Can you work these out from the drawing? Everything is in mm from the part's minimum corner. A direction names the side the tool comes from. Coordinates: 2 decimals unless noted, no trailing zeros. Order: outer loops, then holes, each group sorted by start corner. A loop starts at its lowest first (then second) coordinate and runs counter-clockwise, first axis right, second up. Notation, with made-up numbers: (-28.5, 0) - (23.5, 0) arc R24 ccw to (23.5, 13) - close; hole circle Ø10 at (-3.5, 9.5). An arc over 180 degrees is marked (long way). One line per item, written item: value.
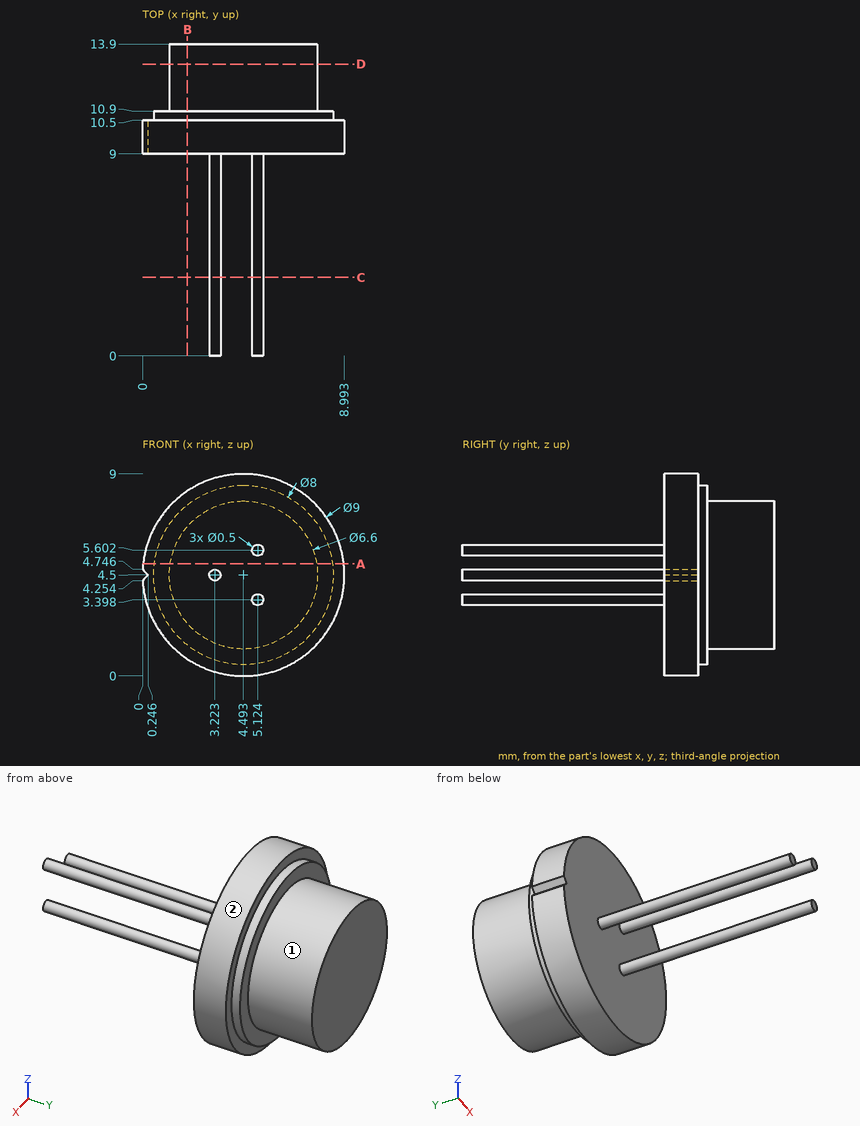
Item 1: For the marked faces 1 and 2, which set-ups out of +Z, -Z, +X, -X, +Y, -Y let a thin tool reach every point of the face, with its end or its side?
Conclusion:
face 1: +Y
face 2: +Y, -Y
Item 2: I want a section at C-C on y = 3.5. Please give me the cut outline in (x, z).
Conclusion:
outline: circle Ø0.5 at (3.22, 4.5); circle Ø0.5 at (5.12, 3.4); circle Ø0.5 at (5.12, 5.6)
Item 3: I want a section at D-D on y = 13. Please give me the cut outline in (x, z).
Conclusion:
outline: circle Ø6.6 at (4.49, 4.5)
Item 4: I want a section at A-A on z = 5. Please give me the cut outline in (x, y) (1 decimal).
Conclusion:
outline: (0, 9) - (9, 9) - (9, 10.5) - (8.5, 10.5) - (8.5, 10.9) - (7.8, 10.9) - (7.8, 13.9) - (1.2, 13.9) - (1.2, 10.9) - (0.5, 10.9) - (0.5, 10.5) - (0, 10.5) - close
Item 5: If I drill on probe 1 along Y at (x, z) = (3.5, 4.75); probe 2 along Y at (x, z) = (3.75, 0.5); probe 3 along Z at (x, y) = (5, 8) (1 decimal), over which ranges is the centre line in solid material (lowest first)?
Conclusion:
probe 1: 9 to 13.9
probe 2: 9 to 10.5
probe 3: 3.2 to 3.6, 5.4 to 5.8
Item 6: I'm going to push flat-ended pins straight in: pin 1 Ø5 at (x, z) = (1.5, 6.5) entering from -Y; pin 2 Ø1 at (x, z) = (7.5, 1.5) entering from +Y; pin 3 Ø1.5 at (y, z) = (2, 8) entering from -X; pin 4 Ø2 at (x, y) = (4.5, 4.5) entering from +Z. Where does each tip first touch, or does it pass through?
Conclusion:
pin 1: y = 0
pin 2: y = 10.9
pin 3: through
pin 4: z = 5.85
Item 7: I want a section at B-B on x = 2. Please give me the cut outline in (y, z).
Conclusion:
outline: (9, 0.75) - (10.5, 0.75) - (10.5, 1.37) - (10.9, 1.37) - (10.9, 2.34) - (13.9, 2.34) - (13.9, 6.66) - (10.9, 6.66) - (10.9, 7.63) - (10.5, 7.63) - (10.5, 8.25) - (9, 8.25) - close
